Here's how the part is built. I have some questions about the finished solid (model axes, mm). A direction names the side the tool comes from. Give positions to 0.01 mm unless a question says otherwise; leave off trailing zeros. Loops run counter-clockwise (first coordinate to the right, second up) from the corner with the lowest first, then second, coordinate; pieces in that order, holes last.
Q1. If we section it at D-D (x = 3): Please give me the cut outline in (y, z), plus the area to 3 significant figures.
Q2. For faces 4 (the face through (0, 18, -2)), 5 (the face through (1.293, -1.479, -0.76)), 6 (the face through (0, 36, 0)), which set-ups out of +Z, -Z, +X, -X, +Y, -Y let a thin tool reach every point of the face, with its end or its side?
Q3. Will this pin go through, and if not, where does the flat tip stop? P1, Ø4, axis at x = -2, y = 25, coming from the +Z side.
Q4. We'd pull the mould along Z, two halves only. Please class faces 1 (the face through (-3.233, -1.028, 1.341)), 2 (the face through (0, 0, 0)), 3 (the face through (-2, 1, -2)): +Z half, -Z half, draft (parallel to the pull), parting line (faces both ways), or undercut.
Q5. If we section it at A-A (x = 0): Please give me the cut outline in (y, z).
Q6. If we section it at B-B (y = 19): Please give me the cut outline in (x, z), plus the area to 3 significant figures.
Q7. If we section it at C-C (z = -2.75): Please give me the cut outline in (x, y), plus the area to 3 significant figures.
Q8. I need wall thicknesses on line 1 (Y direction, x = 0.75, z = -2.25); line 2 (X direction, y = 15, z = 0); line 3 (Z direction, x = -1, y = 30). Which ranges of each line are inside material? Lowest first, please.
Autodesk Inventor part; units mm, degrees
ref_plane "YZ Plane" through (0, 0, 0) normal (1, 0, 0) x (0, 1, 0)
ref_plane "XZ Plane" through (0, 0, 0) normal (0, 1, 0) x (-1, 0, 0)
ref_plane "XY Plane" through (0, 0, 0) normal (0, 0, 1) x (1, 0, 0)
sketch "Szkic1" plane through (0, 0, 0) normal (0, 1, 0) x (-1, 0, 0)
  circle A0 centre (0, 0) radius 3.5
  line L0 (0.866, 1.5) -> (1.7321, 0)
  line L1 (1.7321, 0) -> (0.866, -1.5)
  line L2 (0.866, -1.5) -> (-0.866, -1.5)
  line L3 (-0.866, -1.5) -> (-1.7321, 0)
  line L4 (-1.7321, 0) -> (-0.866, 1.5)
  line L5 (-0.866, 1.5) -> (0.866, 1.5)
  circle A1 centre (0, 0) radius 2
  dimension "d0" = 7
  dimension "d1" = 3
  dimension "d12" = 4
extrude "Wyciągnięcie proste1" add sketch "Szkic1" along normal blind 1 contours A0 | L0 L1 L2 L3 L4 L5 | A1
extrude "Wyciągnięcie proste2" add sketch "Szkic1" against normal blind 3 contours A0 | A1
sketch "Szkic2" plane through (0, 1, 0) normal (0, 1, 0) x (1, 0, 0)
  circle A0 centre (0, 0) radius 2
  dimension "d7" = 4
extrude "Wyciągnięcie proste3" add sketch "Szkic2" along normal blind 35
thread "Gwint1"
properties part number "M4x35" material "Aluminum 6061"
Check sheet entries:
1. outline: (-3, -1.8) - (1, -1.8) - (1, 1.8) - (-3, 1.8) - close
1. area: 14.4 mm2
2. face 4: +Y
2. face 5: -Y
2. face 6: +Z, -Z, +X, -X, +Y
3. P1: stops at z = 2
4. face 1: parting line
4. face 2: undercut
4. face 3: draft
5. outline: (-3, -3.5) - (1, -3.5) - (1, -2) - (36, -2) - (36, 2) - (1, 2) - (1, 3.5) - (-3, 3.5) - (-3, 1.5) - (0, 1.5) - (0, -1.5) - (-3, -1.5) - close
6. outline: circle Ø4 at (0, 0)
6. area: 12.6 mm2
7. outline: (-2.17, -3) - (2.17, -3) - (2.17, 1) - (-2.17, 1) - close
7. area: 17.3 mm2
8. line 1: y = -3 to 1
8. line 2: x = -2 to 2
8. line 3: z = -1.73 to 1.73
